Here's how the part is built. I have some questions about the finished solid (model axes, mm). Face numbers are marked on the shaded views. A direction names the side the tool comes from. Give positions to 0.01 mm unless a question says otherwise; leave off trailing zeros. Write each loop counter-clockwise with the first axis right and the second up, starting at its lowest first coordinate (ties: lowest second). Pieces come first, ordered by that corner, then holes. Notation, with made-up numbers: (-16, 80) -> (18, 80) arc R15 ccw to (18, 97) -> close; hole circle Ø2 at (-17, -6.75). An arc over 180 degrees is marked (long way). Return JSON: item names as keys, results as strings.
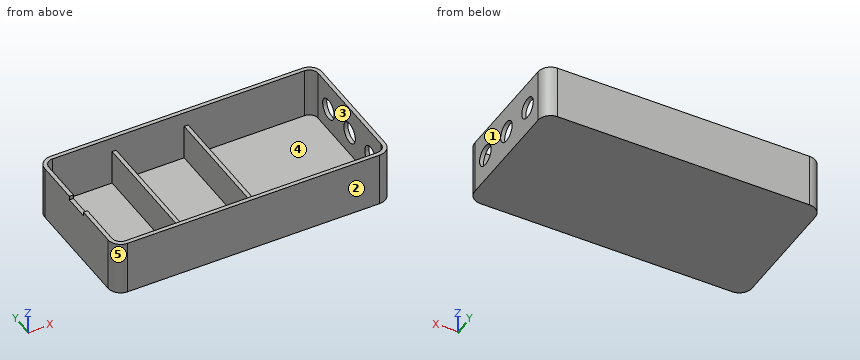
from build123d import *

# Parameters (mm, degrees)
F0_W      = 110
F0_H      = 55
F1_DEPTH  = 21.6
F2_R      = 5
F3_T      = -1.6
F5_W      = 1.6
F5_H      = 51.8
F6_DEPTH  = 14
F7_W      = 10
F7_H      = 1.6
F8_DEPTH  = 1.6
F9_R      = 4.1
F10_DEPTH = 3


with BuildPart() as f1:
    # F0 (on Top) → F1 (new body)
    with BuildSketch(Plane.XY):
        Rectangle(F0_W, F0_H)
    extrude(amount=F1_DEPTH)

    # F2
    f2_edges = [f1.edges().sort_by_distance(p)[0] for p in [
        (-55, -27.5, 10.8),
        (55, -27.5, 10.8),
        (55, 27.5, 10.8),
        (-55, 27.5, 10.8),
    ]]
    fillet(f2_edges, radius=F2_R)

    # F3
    f3_openings = [f1.faces().sort_by_distance(p)[0] for p in [
        (0, 0, 21.6),
    ]]
    offset(amount=F3_T, openings=f3_openings)

    # F5 (on face) → F6 (join)
    with BuildSketch(Plane.XY.offset(1.6)):
        with Locations((-25.6, -0.028194)):
            Rectangle(F5_W, F5_H)
        with Locations((3, -0.028194)):
            Rectangle(F5_W, F5_H)
    extrude(amount=F6_DEPTH)

    # F7 (on face) → F8 (cut, through all)
    with BuildSketch(Plane(origin=(-55, 0, 0), x_dir=(0, -1, 0), z_dir=(-1, 0, 0))):
        with Locations((0, 20.8)):
            Rectangle(F7_W, F7_H)
    extrude(amount=-F8_DEPTH, mode=Mode.SUBTRACT)

    # F9 (on face) → F10 (cut)
    with BuildSketch(Plane.YZ.offset(55)):
        with Locations((0, 10.8)):
            Circle(F9_R)
        with Locations((-15, 10.8)):
            Circle(F9_R)
        with Locations((15, 10.8)):
            Circle(F9_R)
    extrude(amount=-F10_DEPTH, mode=Mode.SUBTRACT)


solid = f1.part
1. Suppose I cut it at D-D, the plane y = 15. List the corners of the cut face in (x, z) for me.
Taken from the geometry:
{"outline": "(-55, 0) -> (55, 0) -> (55, 6.7) -> (53.4, 6.7) -> (53.4, 1.6) -> (3.8, 1.6) -> (3.8, 15.6) -> (2.2, 15.6) -> (2.2, 1.6) -> (-24.8, 1.6) -> (-24.8, 15.6) -> (-26.4, 15.6) -> (-26.4, 1.6) -> (-53.4, 1.6) -> (-53.4, 21.6) -> (-55, 21.6) -> close; (53.4, 14.9) -> (55, 14.9) -> (55, 21.6) -> (53.4, 21.6) -> close"}
2. If I drill on line 1 (X direction, y = 21.5, z = 4.25); line 2 (X direction, y = -1, z = 11.5); line 3 (X direction, y = 21, z = 19.75), over which ranges is the centre line in solid material (lowest first)? Write a range as [from, to].
Taken from the geometry:
{"line 1": "x = [-55, -53.4], [-26.4, -24.8], [2.2, 3.8], [53.4, 55]", "line 2": "x = [-55, -53.4], [-26.4, -24.8], [2.2, 3.8]", "line 3": "x = [-55, -53.4], [53.4, 55]"}
3. Suppose I cut it at B-B, the plane x = -30.5. List the corners of the cut face in (y, z) for me, and give its area (3 significant figures).
Taken from the geometry:
{"outline": "(-27.5, 0) -> (27.5, 0) -> (27.5, 21.6) -> (25.9, 21.6) -> (25.9, 1.6) -> (-25.9, 1.6) -> (-25.9, 21.6) -> (-27.5, 21.6) -> close", "area": "152 mm²"}
4. Suppose I cut it at A-A, the plane y = 0. List the corners of the cut face in (x, z) for me.
Taken from the geometry:
{"outline": "(-55, 0) -> (55, 0) -> (55, 6.7) -> (53.4, 6.7) -> (53.4, 1.6) -> (3.8, 1.6) -> (3.8, 15.6) -> (2.2, 15.6) -> (2.2, 1.6) -> (-24.8, 1.6) -> (-24.8, 15.6) -> (-26.4, 15.6) -> (-26.4, 1.6) -> (-53.4, 1.6) -> (-53.4, 20) -> (-55, 20) -> close; (53.4, 14.9) -> (55, 14.9) -> (55, 21.6) -> (53.4, 21.6) -> close"}
5. Suppose I cut it at C-C, the plane z = 18.25. List the corners of the cut face in (x, y) for me, and give its area (3 significant figures).
Taken from the geometry:
{"outline": "(-55, -22.5) arc R5 ccw to (-50, -27.5) -> (50, -27.5) arc R5 ccw to (55, -22.5) -> (55, 22.5) arc R5 ccw to (50, 27.5) -> (-50, 27.5) arc R5 ccw to (-55, 22.5) -> close; hole (-53.4, -22.5) arc R3.4 ccw to (-50, -25.9) -> (50, -25.9) arc R3.4 ccw to (53.4, -22.5) -> (53.4, 22.5) arc R3.4 ccw to (50, 25.9) -> (-50, 25.9) arc R3.4 ccw to (-53.4, 22.5) -> close", "area": "506 mm²"}
6. If we mould it in two halves opening along Y, with no side actions, what happens to the marked faces 1, 2 and 3? For each: released by +Y, released by -Y, zero draft, split by the parting line, or undercut.
Taken from the geometry:
{"face 1": "zero draft", "face 2": "released by -Y", "face 3": "undercut"}
7. For pin 1 Ø8 at (x, y) = (23, 12.5) entering from +Z; pin 2 Ø0.8 at (x, y) = (3.5, -6) entering from +Z; pin 3 Ø1.3 at (x, z) = (-54, 21) entering from -Y, each with a flat end and sliding along its axis, tell me the tip position at first contact or that it passes through.
Taken from the geometry:
{"pin 1": "stops at z = 1.6", "pin 2": "stops at z = 15.6", "pin 3": "stops at y = -26.21"}
8. Which directions (+Z, -Z, +X, -X, +Y, -Y) give clear straight access to the entire face, cutting with the end or side of a thin tool? Please do the marked faces 4 and 5.
Taken from the geometry:
{"face 4": "+Z", "face 5": "+Z, -Z, -X, -Y"}
